Design review of the part built by this model. Coordinates are the model's own, in mm. Face numbers are marked on the shaded views. A direction names the side the tool comes from. Give positions to 0.01 mm unless a question says otherwise; leave off trailing zeros. Write each loop counter-clockwise with the first axis right and the second up, starting at its lowest first coordinate (ties: lowest second). Pieces come first, ordered by that corner, then holes. Notation, with made-up numbers: M 72,6.25 L 99,6.25 A13 ccw 99,23.25 Z; hole C 79.5,81.5 d2. An arc over 180 degrees is marked long. One line per item, written item: value. Start each with the question number.
```python
from build123d import *

# Parameters (mm, degrees)
F0_R     = 18.5
F1_DEPTH = 20
F2_R     = 14.5
F3_DEPTH = 10
F4_R     = 1


with BuildPart() as f1:
    # F0 (on Top) → F1 (new body)
    with BuildSketch(Plane.XY):
        Circle(F0_R)
    extrude(amount=F1_DEPTH)

    # F2 (on face) → F3 (cut)
    with BuildSketch(Plane.XY.offset(20)):
        Circle(F2_R)
    extrude(amount=-F3_DEPTH, mode=Mode.SUBTRACT)

    # F4
    f4_edges = [f1.edges().sort_by_distance(p)[0] for p in [
        (-18.5, 0, 20),
        (-14.5, 0, 20),
        (-18.5, 0, 0),
        (-14.5, 0, 10),
    ]]
    fillet(f4_edges, radius=F4_R)


solid = f1.part
```
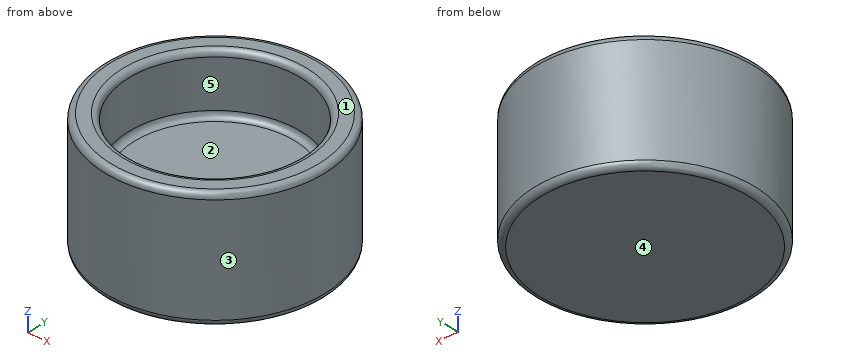
Q1. Take a section at D-D, the plane z = 13.25. Give the boundary of the cut face in (x, y).
Q2. The part is to be moulded in two halves that separate along X. For the marked faces 1, 2 and 3, say which applies: pulls with the +X half, pulls with the -X half, needs draft (parallel to the pull), parting line crosses it, or undercut.
Q3. For P1, Ø6, axis at y = -12.5, z = 8.5, coming from the -X side; P2, Ø10, axis at x = -14.5, z = 6, coming from the -Y side; P3, Ø5, axis at y = 14, z = 12, coming from the +X side; P4, Ø12, axis at x = 13.5, y = -12, coming from the +Z side, all flat-tipped, find the tip position at first contact; note any pin that passes through.
Q4. Wall thickness on line 1 (Y direction, x = 0, z = 16.5); line 2 (Z direction, x = 1, y = 5.5); line 3 (X direction, y = -0.5, z = 12): over which ranges is each line inside the solid? List them lowest first. Write a range as from..to.
Q5. Take a section at C-C, the plane z = 8.25. Give the boundary of the cut face in (x, y), then the cut area to 3 significant figures.
Q6. Take a section at A-A, the plane x = 0. Give the boundary of the cut face in (y, z), then the cut area to 3 significant figures.
Q7. Machinability: for the marked faces 4 and 5, which of the approach directions +Z, -Z, +X, -X, +Y, -Y give a long, thin tool a straight path to every point of the face, cutting with its end or side? Answer none if there is none.
Results list:
1. outline: C 0,0 d37; hole C 0,0 d29
2. face 1: needs draft
2. face 2: undercut
2. face 3: parting line crosses it
3. P1: stops at x = -15.87
3. P2: stops at y = -15.87
3. P3: stops at x = 14.49
3. P4: stops at z = 20
4. line 1: y = -18.5..-14.5, 14.5..18.5
4. line 2: z = 0..10
4. line 3: x = -18.49..-14.49, 14.49..18.49
5. outline: C 0,0 d37
5. area: 1,080 mm^2
6. outline: M -18.5,1 A1 ccw -17.5,0 L 17.5,0 A1 ccw 18.5,1 L 18.5,19 A1 ccw 17.5,20 L 15.5,20 A1 ccw 14.5,19 L 14.5,11 A1 cw 13.5,10 L -13.5,10 A1 cw -14.5,11 L -14.5,19 A1 ccw -15.5,20 L -17.5,20 A1 ccw -18.5,19 Z
6. area: 449 mm^2
7. face 4: -Z, +X, -X, +Y, -Y
7. face 5: +Z
